from build123d import *

# Parameters (mm, degrees)
SKETCH1_R           = 55.5
BOSS_EXTRUDE1_DEPTH = 16
SKETCH2_R           = 12
CUT_EXTRUDE1_DEPTH  = 16
SKETCH3_R           = 2.5
CUT_EXTRUDE2_DEPTH  = 16
SHELL2_OUTLINE_R    = 5.6
SHELL2_DEPTH        = 12.9


# Read off the part's stored shape, not the designer's step: Shell2
with BuildPart() as part:
    # Sketch1 → Boss-Extrude1 (new body)
    with BuildSketch(Plane.XY):
        Circle(SKETCH1_R)
    extrude(amount=BOSS_EXTRUDE1_DEPTH)

    # Sketch2 → Cut-Extrude1 (cut)
    with BuildSketch(Plane.XY.offset(16)):
        with Locations((0, -38)):
            Circle(SKETCH2_R)
    extrude(amount=-CUT_EXTRUDE1_DEPTH, mode=Mode.SUBTRACT)

    # Sketch3 → Cut-Extrude2 (cut)
    with BuildSketch(Plane.XY.offset(16)):
        Circle(SKETCH3_R)
    extrude(amount=-CUT_EXTRUDE2_DEPTH, mode=Mode.SUBTRACT)

    # Shell2 outline → Shell2 (cut)
    with BuildSketch(Plane.XY):
        with BuildLine():
            ThreePointArc((5.329299818, -52.128289474), (0, 52.4), (-5.329299818, -52.128289474))
            ThreePointArc((-5.329299818, -52.128289474), (0, -22.9), (5.329299818, -52.128289474))
        make_face()
        Circle(SHELL2_OUTLINE_R, mode=Mode.SUBTRACT)
    extrude(amount=SHELL2_DEPTH, mode=Mode.SUBTRACT)


solid = part.part
Source: CAD feature listing. Evaluate the final solid. Frame: model axes, mm. A direction names the side the tool comes from. Coordinates: 2 decimals unless noted, no trailing zeros. Loops run counter-clockwise (first coordinate to the right, second up) from the corner with the lowest first, then second, coordinate; pieces in that order, holes last. Notation, with made-up numbers: (61.5, 25) - (70.5, 25) arc R22 cw to (70.5, 49) - close; hole circle Ø11 at (-38, 17). An arc over 180 degrees is marked (long way). One line per item, written item: value. Start each with the question number.
1. Ray query, L1, parallel to Y at x = 0, z = 4.25; L2, parallel to X at y = -39, z = 10.75; L3, parallel to X at y = -29.5, z = 4.25. Return the intervals inside material, ascending.
2. Set-up query: faces 1 (the flat face through (-1, 12, 12.9)), 2 (the cylindrical face through (-1.56, -26.1, 8.11)). Return all of +Z, -Z, +X, -X, +Y, -Y with unobstructed straight access to the full face (end or side cutting, diameter ignored); none if empty.
3. Mould query, pull axis Y, two halves, no side actions, for faces 3 (the cylindrical face through (52.937, 16.671, 7.888)), 4 (the flat face through (0, -24, 0)), 5 (the cylindrical face through (-5.595, 0.246, 6.36)). Classes: pulls with the +Y half, pulls with the -Y half, needs draft (parallel to the pull), parting line crosses it, or undercut.
4. Section B-B (y = 0). Return the cut outline in (x, z), and give its area (3 significant figures).
5. Section D-D (y = -47.5). Return the cut outline in (x, z), and give its area (3 significant figures).
6. Section A-A (x = 0). Return the cut outline in (y, z).
7. Contact query for flat-ended pins moving along their axis: P1, Ø3, axis at y = 31.5, z = 4, coming from the +X side; P2, Ø14.5, axis at x = 0, y = -38, coming from the +Z side; P3, Ø1.5, axis at x = -18.5, z = 5.5, coming from the +Y side; P4, Ø8, axis at y = -29, z = 8.5, coming from the -X side. Output: stop coordinate, or through.
8. Section C-C (z = 7.25). Return the cut outline in (x, y), and give its area (3 significant figures).
Verdict:
1. L1: y = -55.5 to -50, -26 to -22.9, -5.6 to -2.5, 2.5 to 5.6, 52.4 to 55.5
1. L2: x = -39.49 to -35, -15.07 to -11.96, 11.96 to 15.07, 35 to 39.49
1. L3: x = -47.01 to -43.31, -12.48 to -8.47, 8.47 to 12.48, 43.31 to 47.01
2. face 1: -Z
2. face 2: +Z, -Z
3. face 3: parting line crosses it
3. face 4: needs draft
3. face 5: undercut
4. outline: (-55.5, 0) - (-52.4, 0) - (-52.4, 12.9) - (-5.6, 12.9) - (-5.6, 0) - (-2.5, 0) - (-2.5, 16) - (-55.5, 16) - close; (2.5, 0) - (5.6, 0) - (5.6, 12.9) - (52.4, 12.9) - (52.4, 0) - (55.5, 0) - (55.5, 16) - (2.5, 16) - close
4. area: 489 mm2
5. outline: (-28.71, 0) - (-22.12, 0) - (-22.12, 12.9) - (-11.74, 12.9) - (-11.74, 0) - (-7.33, 0) - (-7.33, 16) - (-28.71, 16) - close; (7.33, 0) - (11.74, 0) - (11.74, 12.9) - (22.12, 12.9) - (22.12, 0) - (28.71, 0) - (28.71, 16) - (7.33, 16) - close
5. area: 416 mm2
6. outline: (-55.5, 0) - (-50, 0) - (-50, 16) - (-55.5, 16) - close; (-26, 0) - (-22.9, 0) - (-22.9, 12.9) - (-5.6, 12.9) - (-5.6, 0) - (-2.5, 0) - (-2.5, 16) - (-26, 16) - close; (2.5, 0) - (5.6, 0) - (5.6, 12.9) - (52.4, 12.9) - (52.4, 0) - (55.5, 0) - (55.5, 16) - (2.5, 16) - close
7. P1: stops at x = 46.69
7. P2: passes through
7. P3: stops at y = 52.59
7. P4: stops at x = -49.55
8. outline: circle Ø111 at (0, 0); circle Ø11.2 at (0, 0); hole circle Ø24 at (0, -38); hole (-5.33, -52.13) arc R15.1 cw (long way) to (5.33, -52.13) arc R52.4 ccw (long way) to start; hole circle Ø5 at (0, 0)
8. area: 1,390 mm2
